Check sheet for the modelled part. Datum: model origin and axes. Units: mm. A direction names the side the tool comes from. Round coordinates to 2 decimals unless told otherwise and drop trailing zeros. Order: outer loops, then holes, each group sorted by start corner. A loop starts at its lowest first (then second) coordinate and runs counter-clockwise, first axis right, second up.
(1) Sectioned sample at B-B, the plane x = 10.5. Enter the section's corners in (y, z), and give its area (3 significant figures).
(2) Tool access check on faces 5 (the flat face through (-41, 6.25, 1)), 6 (the flat face through (39.8, 3, 1)), 7 (the flat face through (45, 1, 1)). Record the directions out of +Z, -Z, +X, -X, +Y, -Y that give a thin tool (end or side, any length) a straight path to the whole face; none if there is none.
(3) Depth check by flat-ended pin: pin 1 (1.8 mm diameter, centred on x = 10.5, y = 6.25, fed in from +Z). Enter the tip coordinate at first touch or a pass-through.
(4) Mould release check, pull along X, two halves, no side actions. Record for faces 1 (the cylindrical face through (32.55, -5.92, 1.48)), 2 (the cylindrical face through (-44.248, -8.037, 1.521)), 3 (the flat face through (-42, 8.75, 1)), 4 (the flat face through (-39.8, 3, 1)): released by +X, released by -X, zero draft, split by the parting line, or undercut.
(5) Sectioned sample at C-C, the plane z = 1.55. Count the separate pieces of the cut face and the enclosed holes in it, and give its area (3 significant figures).
(6) Thickness scan on probe 1 along Y at (x, z) = (-10.5, 0.6); probe 2 along X at (y, z) = (8.25, 1.15); probe 3 along X at (y, z) = (-5.5, 1.45). Record the ranges inside material, lowest first.
(7) Sectioned sample at A-A, the plane y = 2.5. Enter the section's corners in (x, z), and give its area (3 significant figures).
```python
from build123d import *

# Parameters (mm, degrees)
SKETCH1_R           = 1.1
BOSS_EXTRUDE1_DEPTH = 3
FILLET1_R           = 2.5


with BuildPart() as part:
    # Sketch1 → Boss-Extrude1 (new body)
    with BuildSketch(Plane.XY):
        Polygon((-45, -8.75), (45, -8.75), (45, 8.75), (39.8, 8.75), (39.8, 6.25), (42.3, 6.25), (42.3, 4.25), (39.8, 4.25), (39.8, 1.75), (37.6, 1.75), (37.6, 4.25), (35.1, 4.25), (35.1, 6.25), (37.6, 6.25), (37.6, 8.75), (-37.6, 8.75), (-37.6, 6.25), (-35.1, 6.25), (-35.1, 4.25), (-37.6, 4.25), (-37.6, 1.75), (-39.8, 1.75), (-39.8, 4.25), (-42.3, 4.25), (-42.3, 6.25), (-39.8, 6.25), (-39.8, 8.75), (-45, 8.75), align=None)
        with Locations((-10.5, 6.25)):
            Circle(SKETCH1_R, mode=Mode.SUBTRACT)
        with Locations(Location((-10.5, -6.25, 0), (0, 0, 180))):
            Circle(SKETCH1_R, mode=Mode.SUBTRACT)
        with Locations((10.5, -6.25)):
            Circle(SKETCH1_R, mode=Mode.SUBTRACT)
        with Locations(Location((10.5, 6.25, 0), (0, 0, 180))):
            Circle(SKETCH1_R, mode=Mode.SUBTRACT)
        with Locations((-31.5, 6.25)):
            Circle(SKETCH1_R, mode=Mode.SUBTRACT)
        with Locations(Location((-31.5, -6.25, 0), (0, 0, 180))):
            Circle(SKETCH1_R, mode=Mode.SUBTRACT)
        with Locations((31.5, -6.25)):
            Circle(SKETCH1_R, mode=Mode.SUBTRACT)
        with Locations(Location((31.5, 6.25, 0), (0, 0, 180))):
            Circle(SKETCH1_R, mode=Mode.SUBTRACT)
    extrude(amount=BOSS_EXTRUDE1_DEPTH)

    # Fillet1
    fillet1_edges = [part.edges().sort_by_distance(p)[0] for p in [
        (45, -8.75, 1.5),
        (-45, -8.75, 1.5),
    ]]
    fillet(fillet1_edges, radius=FILLET1_R)


solid = part.part
```
Derived:
1. outline: (-8.75, 0) - (-7.35, 0) - (-7.35, 3) - (-8.75, 3) - close; (-5.15, 0) - (5.15, 0) - (5.15, 3) - (-5.15, 3) - close; (7.35, 0) - (8.75, 0) - (8.75, 3) - (7.35, 3) - close
1. area: 39.3 mm2
2. face 5: +Z, -Z
2. face 6: +Z, -Z, +Y
2. face 7: +Z, -Z, +X, +Y, -Y
3. pin 1: passes through
4. face 1: undercut
4. face 2: released by -X
4. face 3: zero draft
4. face 4: undercut
5. separate pieces: 1
5. enclosed holes: 8
5. area: 1,490 mm2
6. probe 1: y = -8.75 to -7.35, -5.15 to 5.15, 7.35 to 8.75
6. probe 2: x = -45 to -39.8, -37.6 to 37.6, 39.8 to 45
6. probe 3: x = -45 to -32.3, -30.7 to -11.3, -9.7 to 9.7, 11.3 to 30.7, 32.3 to 45
7. outline: (-45, 0) - (-39.8, 0) - (-39.8, 3) - (-45, 3) - close; (-37.6, 0) - (37.6, 0) - (37.6, 3) - (-37.6, 3) - close; (39.8, 0) - (45, 0) - (45, 3) - (39.8, 3) - close
7. area: 257 mm2
